Build history of the part. All positions in model axes, mm. A direction names the side the tool comes from. Give positions to 0.01 mm unless a question says otherwise; leave off trailing zeros. Write each loop counter-clockwise with the first axis right and the second up, starting at its lowest first coordinate (ties: lowest second). Pieces come first, ordered by that corner, then holes. Notation, with made-up numbers: (-31, 23.25) -> (13, 23.25) arc R10 ccw to (13, 40.25) -> close; hole circle Ø10 at (46, 35). An arc over 180 degrees is marked (long way). Write item = value, one per line. Start each with the question number.
Q1. Saw through at B-B, the plane x = 41.5. List the corners of the cut face in (y, z).
Q2. Drop flat-ended pins along their axis: P1, Ø4, axis at x = 47, z = 8.5, coming from the +Y side; P2, Ø3, axis at x = 8.07, z = 6.35, coming from the +Y side; P3, Ø6, axis at x = 32, z = 9, coming from the +Y side; P4, Ø5, axis at y = 18, z = 8.5, coming from the +X side. Give the stop position or say it passes through.
Q3. Saw through at A-A, the plane z = 6.35. List the corners of the cut face in (x, y), then the cut area to 3 significant figures.
Q4. Mould opens along Z. For faces 1 (the face through (17, 15, 0)), 2 (the face through (25.064, 23.926, 6.261)), 3 (the face through (10.34, 0.39, 7.07)) say: pulls with the +Z half, pulls with the -Z half, needs draft (parallel to the pull), parting line crosses it, or undercut.
Q5. Saw through at D-D, the plane x = 19. List the corners of the cut face in (y, z), then the cut area to 3 significant figures.
Q6. Wall check: line 1 (Y direction, x = 6, z = 1.75); line 2 (Y direction, x = 25, z = 10.5); line 3 (X direction, y = 13.75, z = 4.75). Give the ranges that are in metal, low to high.
Q7. Saw through at C-C, the plane y = 19.75. List the corners of the cut face in (x, z).
Q8. Tool access for faces 4 (the face through (45, 0.794, 8)), 5 (the face through (17, 15, 12.7)), 6 (the face through (16.62, 8.53, 6.26)), 7 (the face through (1.61, 0.391, 11.135)), 8 (the face through (5.5, 0.794, 6.3)): list every direction of +Z, -Z, +X, -X, +Y, -Y with a clear straight run to the whole face (end or side of a thin tool).
Autodesk Inventor part; units mm, degrees
ref_plane "YZ Plane" through (0, 0, 0) normal (1, 0, 0) x (0, 1, 0)
ref_plane "XZ Plane" through (0, 0, 0) normal (0, 1, 0) x (-1, 0, 0)
ref_plane "XY Plane" through (0, 0, 0) normal (0, 0, 1) x (1, 0, 0)
sketch "Sketch1" plane through (0, 0, 0) normal (0, 0, 1) x (1, 0, 0)
  line L0 (0, 0) -> (14.4203, 0)
  line L1 (16.0018, 1.4491) -> (17.2586, 15.8146)
  arc A0 (33.2345, 15.8146) -> (17.2586, 15.8146) centre (25.2465, 15.1157) ccw
  line L2 (33.2345, 15.8146) -> (34.4913, 1.4491)
  line L3 (36.0728, 0) -> (50.4931, 0)
  arc A1 (14.4203, 0) -> (16.0018, 1.4491) centre (14.4203, 1.5875) ccw
  arc A2 (34.4913, 1.4491) -> (36.0728, 0) centre (36.0728, 1.5875) ccw
  line L4 (0, 0.7937) -> (14.4203, 0.7937)
  arc A3 (14.4203, 0.7937) -> (15.2111, 1.5183) centre (14.4203, 1.5875) ccw
  line L5 (15.2111, 1.5183) -> (16.4679, 15.8838)
  arc A4 (34.0252, 15.8838) -> (16.4679, 15.8838) centre (25.2465, 15.1157) ccw
  line L6 (34.0252, 15.8838) -> (35.282, 1.5183)
  arc A5 (35.282, 1.5183) -> (36.0728, 0.7938) centre (36.0728, 1.5875) ccw
  line L7 (36.0728, 0.7938) -> (50.4931, 0.7938)
  line L8 (0, 0.7937) -> (0, 0)
  line L9 (50.4931, 0.7938) -> (50.4931, 0)
  line L10 (17.944, 18.4277) -> (32.549, 18.4277) construction
  point P0 (15.875, 0)
  dimension "d0" = 15.875
  dimension "d1" = 15.875
  dimension "d2" = 1.5875
  dimension "d3" = 95
  dimension "d4" = 95
  dimension "d6" = 0.7937
  dimension "d18" = 14.605
  dimension "d19" = 18.4277
extrude "Extrusion1" add sketch "Sketch1" along normal blind 12.7
chamfer "Chamfer1" distance 3.175 angle 45 4 edges at (0, 0.3969, 12.7) (50.4931, 0.3969, 12.7) (50.4931, 0.3969, 0) (0, 0.3969, 0)
sketch "Sketch2" plane through (36.0728, 0, 0) normal (0, -1, 0) x (1, 0, 0)
  line L0 (0, 12.7) -> (11.2453, 12.7)
  line L1 (0, 0) -> (0, 12.7)
  line L2 (0, 0) -> (11.2453, 0)
  line L3 (-32.8978, 0) -> (-36.0728, 3.175)
  line L4 (-32.8978, 0) -> (-21.6524, 0)
  line L5 (-21.6524, 0) -> (-21.6524, 12.7)
  line L6 (-32.8978, 12.7) -> (-21.6524, 12.7)
  line L7 (-36.0728, 9.525) -> (-32.8978, 12.7)
  line L8 (-36.0728, 3.175) -> (-36.0728, 9.525)
  line L9 (6.35, 12.7) -> (6.35, 0) construction
  line L10 (-28.0024, 12.7) -> (-28.0024, 0) construction
  circle A0 centre (-28.0024, 6.35) radius 2.3813
  circle A1 centre (6.35, 6.35) radius 2.3813
  point P0 (-36.0728, 0)
  dimension "d12" = 4.7625
  dimension "d13" = 4.7625
  dimension "d14" = 6.35
  dimension "d15" = 6.35
extrude "Extrusion2" cut sketch "Sketch2" against normal through all contours A0 | A1
equation "\"d4\" = d3"
equation "\"d12\" = d13"
equation "\"d15\" = d14"
properties part number "Pneumatics Steel Bracket" material "Steel"
Report:
q1.outline = (0, 0) -> (0.79, 0) -> (0.79, 4.15) -> (0, 4.15) -> close; (0, 8.55) -> (0.79, 8.55) -> (0.79, 12.7) -> (0, 12.7) -> close
q2.P1 = 0.79
q2.P2 = through
q2.P3 = 23.09
q2.P4 = 34.06
q3.outline = (0, 0) -> (5.69, 0) -> (5.69, 0.79) -> (0, 0.79) -> close; (10.45, 0) -> (14.42, 0) arc R1.59 ccw to (16, 1.45) -> (17.26, 15.81) arc R8.02 cw to (33.23, 15.81) -> (34.49, 1.45) arc R1.59 ccw to (36.07, 0) -> (40.04, 0) -> (40.04, 0.79) -> (36.07, 0.79) arc R0.79 cw to (35.28, 1.52) -> (34.03, 15.88) arc R8.81 ccw to (16.47, 15.88) -> (15.21, 1.52) arc R0.79 cw to (14.42, 0.79) -> (10.45, 0.79) -> close; (44.8, 0) -> (50.49, 0) -> (50.49, 0.79) -> (44.8, 0.79) -> close
q3.area = 60.8 mm2
q4.face_1 = pulls with the -Z half
q4.face_2 = needs draft
q4.face_3 = undercut
q5.outline = (20.14, 0) -> (21.33, 0) -> (21.33, 12.7) -> (20.14, 12.7) -> close
q5.area = 15.1 mm2
q6.line_1 = 0 to 0.79
q6.line_2 = 23.13 to 23.92
q6.line_3 = 16.28 to 17.08, 33.42 to 34.21
q7.outline = (17.75, 0) -> (18.7, 0) -> (18.7, 12.7) -> (17.75, 12.7) -> close; (31.79, 0) -> (32.74, 0) -> (32.74, 12.7) -> (31.79, 12.7) -> close
q8.face_4 = +Z, -Z, +X, +Y
q8.face_5 = +Z, +X, -X, +Y, -Y
q8.face_6 = +Z, -Z, -Y
q8.face_7 = +Z, -X, +Y, -Y
q8.face_8 = +Z, -Z, -X, +Y
